Input: part model. Units: mm. Frame: model coordinates. A direction names the side the tool comes from. Give positions to 0.01 mm unless a question says otherwise; leave off trailing zeros. Loops run counter-clockwise (first coordinate to the right, second up) from the corner with the lowest first, then second, coordinate; pieces in that order, holes last. Notation, with made-up numbers: (22, -12) - (63, -12) arc R23 cw to (63, 24) - close; hole circle Ø2 at (-1.5, 88). An arc over 180 degrees is marked (long way). Answer as a JSON object with one key per item and string values. Group by question number.
(1) Section query D-D (z = -5). Return loops of the section in (x, y).
(2) Material intervals for L1, parallel to Y at x = -3.5, z = 5; L2, parallel to Z at x = 3.75, y = 57; L3, parallel to X at y = -10, z = -1.25, sorted ascending.
(3) Section query B-B (y = -1). Return loops of the section in (x, z), plus the area to 4 significant figures.
(4) Section query C-C (x = 0.75). Return loops of the section in (y, z).
(5) Section query A-A (y = 57.05). Return loops of the section in (x, z), plus the area to 4 significant figures.
(6) Mould query, pull axis Y, two halves, no side actions, for faces 1 (the flat face through (-7.25, 57, 0)), 2 (the cylindrical face through (-0.1, -8.38, 5.69)), 3 (the flat face through (0, -14.1, -4)). Classes: +Y half, -Y half, draft (parallel to the pull), parting line (faces both ways), or undercut.
(7) Access query for faces 4 (the flat face through (0, -7, 8.5)), 5 (the flat face through (0, -7, -8.5)), 6 (the flat face through (0, 57, -8.5)), 7 (the flat face through (-5, -7, 0)), 8 (the flat face through (0, 50, 0)). Directions: +Z, -Z, +X, -X, +Y, -Y. A direction counts if a zero-diameter tool reaches every point of the face in a straight line with its end or side. Return the directions, or none.
(8) Pin query (flat end, axial travel): P1, Ø6.5, axis at x = 0.5, y = -4, coming from the -Z side; P2, Ø3, axis at x = 7.5, z = 7, coming from the -Y side; P3, Ø1.5, axis at y = 57.5, z = 0, coming from the -X side; P4, Ø6, axis at x = -2.5, y = -4.5, coming from the +Z side. Return the tip coordinate at first contact, or that it passes through.
```python
from build123d import *

# Parameters (mm, degrees)
SKETCH1_W             = 20
SKETCH1_H             = 20
BOSS_EXTRUDE1_DEPTH   = 50
BOSS_EXTRUDE2_DEPTH   = 39.1
CUT_EXTRUDE1_DEPTH    = 14.1
CUT_EXTRUDE2_START    = -14.1
CUT_EXTRUDE2_DEPTH    = 14.1
M3X0_5_TAPPED_HOLE1_D = 3
FILLET1_R             = 1


with BuildPart() as part:
    # Sketch1 → Boss-Extrude1 (new body)
    with BuildSketch(Plane(origin=(0, 0, 0), x_dir=(1, 0, 0), z_dir=(0, 1, 0))):
        Rectangle(SKETCH1_W, SKETCH1_H)
    extrude(amount=BOSS_EXTRUDE1_DEPTH)

    # Sketch2 → Boss-Extrude2 (add, symmetric)
    with BuildSketch(Plane(origin=(0, 25, 0), x_dir=(1, 0, 0), z_dir=(0, 1, 0))):
        with BuildLine():
            Line((-6.25, -8.5), (6.25, -8.5))
            ThreePointArc((6.25, -8.5), (6.957106781, -8.207106781), (7.25, -7.5))
            Line((7.25, -7.5), (7.25, 7.5))
            ThreePointArc((7.25, 7.5), (6.957106781, 8.207106781), (6.25, 8.5))
            Line((6.25, 8.5), (-6.25, 8.5))
            ThreePointArc((-6.25, 8.5), (-6.957106781, 8.207106781), (-7.25, 7.5))
            Line((-7.25, 7.5), (-7.25, -7.5))
            ThreePointArc((-7.25, -7.5), (-6.957106781, -8.207106781), (-6.25, -8.5))
        make_face()
    extrude(amount=BOSS_EXTRUDE2_DEPTH, both=True)

    # Sketch3 → Cut-Extrude1 (cut)
    with BuildSketch(Plane(origin=(0, 64.1, 0), x_dir=(1, 0, 0), z_dir=(0, 1, 0))):
        with BuildLine():
            Line((-4, -2.5), (4, -2.5))
            ThreePointArc((4, -2.5), (4.707106781, -2.207106781), (5, -1.5))
            Line((5, -1.5), (5, 1.5))
            ThreePointArc((5, 1.5), (4.707106781, 2.207106781), (4, 2.5))
            Line((4, 2.5), (-4, 2.5))
            ThreePointArc((-4, 2.5), (-4.707106781, 2.207106781), (-5, 1.5))
            Line((-5, 1.5), (-5, -1.5))
            ThreePointArc((-5, -1.5), (-4.707106781, -2.207106781), (-4, -2.5))
        make_face()
    extrude(amount=-CUT_EXTRUDE1_DEPTH, mode=Mode.SUBTRACT)

    # Sketch4 → Cut-Extrude2 (cut)
    with BuildSketch(Plane.XZ.offset(14.1).offset(CUT_EXTRUDE2_START)):
        with BuildLine():
            Line((-4, -2.5), (4, -2.5))
            ThreePointArc((4, -2.5), (4.707106781, -2.207106781), (5, -1.5))
            Line((5, -1.5), (5, 1.5))
            ThreePointArc((5, 1.5), (4.707106781, 2.207106781), (4, 2.5))
            Line((4, 2.5), (-4, 2.5))
            ThreePointArc((-4, 2.5), (-4.707106781, 2.207106781), (-5, 1.5))
            Line((-5, 1.5), (-5, -1.5))
            ThreePointArc((-5, -1.5), (-4.707106781, -2.207106781), (-4, -2.5))
        make_face()
    extrude(amount=CUT_EXTRUDE2_DEPTH, mode=Mode.SUBTRACT)

    # M3x0.5 Tapped Hole1 (through all)
    with Locations(Plane(origin=(7.25, 0, 0), x_dir=(0, 0, -1), z_dir=(1, 0, 0))):
        with Locations((5, 57.05), (5, -7.05), (-5, 57.05), (-5, -7.05)):
            Hole(M3X0_5_TAPPED_HOLE1_D / 2)

    # Fillet1
    fillet1_edges = [part.edges().sort_by_distance(p)[0] for p in [
        (10, 25, 10),
        (-10, 25, 10),
        (-10, 25, -10),
        (10, 25, -10),
    ]]
    fillet(fillet1_edges, radius=FILLET1_R)


solid = part.part
```
Recorded:
{
 "1": {"outline": "(-10, 0) - (-7.25, 0) - (-7.25, -5.55) - (7.25, -5.55) - (7.25, 0) - (10, 0) - (10, 50) - (7.25, 50) - (7.25, 55.55) - (-7.25, 55.55) - (-7.25, 50) - (-10, 50) - close; (-7.25, -14.1) - (7.25, -14.1) - (7.25, -8.55) - (-7.25, -8.55) - close; (-7.25, 58.55) - (7.25, 58.55) - (7.25, 64.1) - (-7.25, 64.1) - close"},
 "2": {"L1": "y = -14.1 to -8.55, -5.55 to 55.55, 58.55 to 64.1", "L2": "z = -8.5 to -6.5, -3.5 to -2.5, 2.5 to 3.5, 6.5 to 8.5", "L3": "x = -7.25 to -5, 5 to 7.25"},
 "3": {"outline": "(-7.25, -7.5) arc R1 ccw to (-6.25, -8.5) - (6.25, -8.5) arc R1 ccw to (7.25, -7.5) - (7.25, 7.5) arc R1 ccw to (6.25, 8.5) - (-6.25, 8.5) arc R1 ccw to (-7.25, 7.5) - close; hole (-5, -1.5) arc R1 ccw to (-4, -2.5) - (4, -2.5) arc R1 ccw to (5, -1.5) - (5, 1.5) arc R1 ccw to (4, 2.5) - (-4, 2.5) arc R1 ccw to (-5, 1.5) - close", "area": "196.5 mm^2"},
 "4": {"outline": "(-14.1, -8.5) - (0, -8.5) - (0, -10) - (50, -10) - (50, -8.5) - (64.1, -8.5) - (64.1, -2.5) - (50, -2.5) - (50, 2.5) - (64.1, 2.5) - (64.1, 8.5) - (50, 8.5) - (50, 10) - (0, 10) - (0, 8.5) - (-14.1, 8.5) - (-14.1, 2.5) - (0, 2.5) - (0, -2.5) - (-14.1, -2.5) - close; hole circle Ø3 at (-7.05, -5); hole circle Ø3 at (-7.05, 5); hole circle Ø3 at (57.05, -5); hole circle Ø3 at (57.05, 5)"},
 "5": {"outline": "(-7.25, -7.5) arc R1 ccw to (-6.25, -8.5) - (6.25, -8.5) arc R1 ccw to (7.25, -7.5) - (7.25, -6.5) - (-7.25, -6.5) - close; (-7.25, -3.5) - (7.25, -3.5) - (7.25, 3.5) - (-7.25, 3.5) - close; (-7.25, 6.5) - (7.25, 6.5) - (7.25, 7.5) arc R1 ccw to (6.25, 8.5) - (-6.25, 8.5) arc R1 ccw to (-7.25, 7.5) - close; hole (-5, -1.5) arc R1 ccw to (-4, -2.5) - (4, -2.5) arc R1 ccw to (5, -1.5) - (5, 1.5) arc R1 ccw to (4, 2.5) - (-4, 2.5) arc R1 ccw to (-5, 1.5) - close", "area": "109.5 mm^2"},
 "6": {"face 1": "draft", "face 2": "undercut", "face 3": "-Y half"},
 "7": {"face 4": "+Z, +X, -X, -Y", "face 5": "-Z, +X, -X, -Y", "face 6": "-Z, +X, -X, +Y", "face 7": "-Y", "face 8": "+Y"},
 "8": {"P1": "stops at z = -8.5", "P2": "stops at y = -14.1", "P3": "stops at x = -7.25", "P4": "stops at z = 8.5"}
}
